Part model, mm, in its own coordinate system. A direction names the side the tool comes from. Round coordinates to 2 decimals unless told otherwise and drop trailing zeros. Loops run counter-clockwise (first coordinate to the right, second up) from the corner with the lowest first, then second, coordinate; pieces in that order, holes last. Notation, with made-up numbers: M 49,46 L 82,46 A18 ccw 82,75 Z; hole C 32,-28 d8. An arc over 180 degrees is marked long. Put each result on its own line as item: value. Start each with the question number.
1) Slice it at D-D on z = -5. Give the cut face in (x, y), then the cut area to 3 significant figures.
2) Drop flat-ended pins along their axis: pin 1 Ø2 at (x, y) = (-0.5, -3) entering from +Z (3 decimals); pin 2 Ø1.5 at (x, y) = (-1.5, -1.5) entering from -Z. Give the stop position or say it passes through.
3) Slice it at B-B on x = 0.25. Give the cut face in (y, z) (3 decimals).
4) Pull direction Z, two halves, no side cores. Call faces 1 (the flat face through (-3.25, -1.7, -0.1)), 2 (the cylindrical face through (0.071, -2.218, 12.774)), 3 (the cylindrical face through (1.949, -1.014, 4.965)): +Z half, -Z half, draft (parallel to the pull), parting line (faces both ways), or undercut.
5) Slice it at A-A on y = -2.5. Give the cut face in (x, z) (3 decimals).
6) Which spindle directions (+Z, -Z, +X, -X, +Y, -Y) get a long thin tool onto all of the face, cutting with end or side? Do faces 4 (the flat face through (0, -3, 6.375)), 5 (the flat face through (2.25, -1, 0)), 6 (the flat face through (0, -4.5, 8)). Say none if no direction does.
7) Slice it at C-C on y = -0.45. Give the cut face in (x, z) (3 decimals), then the cut area to 3 significant figures.
8) Probe line 1 along Z through (x, y) = (0, -2.7) (3 decimals); line 2 along Z through (x, y) = (-1, -3.7) (3 decimals); line 3 along X through (y, z) = (-0.5, -2). List the from-to ranges inside material, lowest first.
```python
from build123d import *

# Parameters (mm, degrees)
SKETCH1_W            = 4.5
SKETCH1_H            = 10.5
BOSS_EXTRUDE1_DEPTH  = 2
BOSS_EXTRUDE2_START  = -2
BOSS_EXTRUDE2_DEPTH  = 2.5
M2_CLEARANCE_HOLE1_D = 2.4
FILLET1_R            = 1


with BuildPart() as part:
    # Sketch1 → Boss-Extrude1 (new body)
    with BuildSketch(Plane(origin=(0, 0, 0), x_dir=(1, 0, 0), z_dir=(0, 1, 0))):
        with BuildLine():
            Line((3.25, 9.525), (3.25, -9.525))
            ThreePointArc((3.25, -9.525), (0, -12.775), (-3.25, -9.525))
            Line((-3.25, -9.525), (-3.25, 9.525))
            ThreePointArc((-3.25, 9.525), (0, 12.775), (3.25, 9.525))
        make_face()
        Rectangle(SKETCH1_W, SKETCH1_H, mode=Mode.SUBTRACT)
    extrude(amount=-BOSS_EXTRUDE1_DEPTH)

    # Sketch1<3> → Boss-Extrude2 (add)
    with BuildSketch(Plane(origin=(0, 0, 0), x_dir=(1, 0, 0), z_dir=(0, 1, 0)).offset(BOSS_EXTRUDE2_START)):
        with BuildLine():
            Line((-3.25, 9.525), (-3.25, 6.375))
            Line((-3.25, 6.375), (3.25, 6.375))
            Line((3.25, 6.375), (3.25, 9.525))
            ThreePointArc((3.25, 9.525), (0, 12.775), (-3.25, 9.525))
        make_face()
        with BuildLine():
            Line((3.25, -6.375), (-3.25, -6.375))
            Line((-3.25, -6.375), (-3.25, -9.525))
            ThreePointArc((-3.25, -9.525), (0, -12.775), (3.25, -9.525))
            Line((3.25, -9.525), (3.25, -6.375))
        make_face()
    extrude(amount=-BOSS_EXTRUDE2_DEPTH)

    # M2 Clearance Hole1 (through all)
    with Locations(Plane(origin=(0, -4.5, 0), x_dir=(-1, 0, 0), z_dir=(0, -1, 0))):
        with Locations((0, 9.525), (0, -9.525)):
            Hole(M2_CLEARANCE_HOLE1_D / 2)

    # Fillet1
    fillet1_edges = [part.edges().sort_by_distance(p)[0] for p in [
        (-2.25, -1, 5.25),
        (2.25, -1, 5.25),
        (2.25, -1, -5.25),
        (-2.25, -1, -5.25),
    ]]
    fillet(fillet1_edges, radius=FILLET1_R)


solid = part.part
```
Recorded:
1. outline: M -3.25,-2 L -1.91,-2 L -1.91,0 L -3.25,0 Z; M 1.91,-2 L 3.25,-2 L 3.25,0 L 1.91,0 Z
1. area: 5.35 mm2
2. pin 1: stops at z = 12.775
2. pin 2: stops at z = -12.69
3. outline: M -4.5,-12.765 L 0,-12.765 L 0,-10.699 L -4.5,-10.699 Z; M -4.5,-8.351 L 0,-8.351 L 0,-5.25 L -2,-5.25 L -2,-6.375 L -4.5,-6.375 Z; M -4.5,6.375 L -2,6.375 L -2,5.25 L 0,5.25 L 0,8.351 L -4.5,8.351 Z; M -4.5,10.699 L 0,10.699 L 0,12.765 L -4.5,12.765 Z
4. face 1: draft
4. face 2: +Z half
4. face 3: undercut
5. outline: M -3.25,-9.525 A3.25 ccw 3.25,-9.525 L 3.25,-6.375 L -3.25,-6.375 Z; M -3.25,6.375 L 3.25,6.375 L 3.25,9.525 A3.25 ccw -3.25,9.525 Z; hole C 0,-9.525 d2.4; hole C 0,9.525 d2.4
6. face 4: +X, -X, -Y
6. face 5: +Y, -Y
6. face 6: +Z, -Z, +X, -X, -Y
7. outline: M -3.25,-9.525 A3.25 ccw 3.25,-9.525 L 3.25,9.525 A3.25 ccw -3.25,9.525 Z; hole M -2.25,-4.25 A1 ccw -1.25,-5.25 L 1.25,-5.25 A1 ccw 2.25,-4.25 L 2.25,4.25 A1 ccw 1.25,5.25 L -1.25,5.25 A1 ccw -2.25,4.25 Z; hole C 0,-9.525 d2.4; hole C 0,9.525 d2.4
7. area: 102 mm2
8. line 1: z = -12.775 to -10.725, -8.325 to -6.375, 6.375 to 8.325, 10.725 to 12.775
8. line 2: z = -12.617 to -10.188, -8.862 to -6.375, 6.375 to 8.862, 10.188 to 12.617
8. line 3: x = -3.25 to -2.25, 2.25 to 3.25
